```python
from build123d import *

# Parameters (mm, degrees)
SKETCH1_R           = 18.5
SKETCH1_R_2         = 11.5
BOSS_EXTRUDE1_DEPTH = 1.6
SKETCH2_W           = 5
SKETCH2_H           = 5
BOSS_EXTRUDE2_DEPTH = 1.7
CIRPATTERN1_COUNT   = 12
SKETCH3_R           = 1
CUT_EXTRUDE1_DEPTH  = 2
CIRPATTERN2_COUNT   = 2
SKETCH4_R           = 1
CUT_EXTRUDE2_DEPTH  = 10
CIRPATTERN3_COUNT   = 2


with BuildPart() as part:
    # Sketch1 → Boss-Extrude1 (new body)
    with BuildSketch(Plane.XY):
        Circle(SKETCH1_R)
        Circle(SKETCH1_R_2, mode=Mode.SUBTRACT)
    extrude(amount=BOSS_EXTRUDE1_DEPTH)

    # Sketch2 → Boss-Extrude2 (add)
    with BuildSketch(Plane.XY.offset(1.6)):
        with Locations((0, 15)):
            Rectangle(SKETCH2_W, SKETCH2_H)
    boss_extrude2 = extrude(amount=BOSS_EXTRUDE2_DEPTH)

    # CirPattern1: Boss-Extrude2 ×12 about axis
    cirpattern1_axis = Axis((0, 0, 0), (0, 0, 1))
    for i in range(1, CIRPATTERN1_COUNT):
        add(boss_extrude2.rotate(cirpattern1_axis, i * 360 / CIRPATTERN1_COUNT))

    # Sketch3 → Cut-Extrude1 (cut)
    with BuildSketch(Plane.XY.offset(1.6)):
        with Locations((-4.270514244, 15.937776134)):
            Circle(SKETCH3_R)
    cut_extrude1 = extrude(amount=-CUT_EXTRUDE1_DEPTH, mode=Mode.SUBTRACT)

    # CirPattern2: Cut-Extrude1 ×2 about axis
    cirpattern2_axis = Axis((0, 0, 0), (0, 0, 1))
    for i in range(1, CIRPATTERN2_COUNT):
        add(cut_extrude1.rotate(cirpattern2_axis, i * 360 / CIRPATTERN2_COUNT), mode=Mode.SUBTRACT)

    # Sketch4 → Cut-Extrude2 (cut)
    with BuildSketch(Plane.XY.offset(1.6)):
        with Locations((-15.937776134, 4.270514244)):
            Circle(SKETCH4_R)
    cut_extrude2 = extrude(amount=-CUT_EXTRUDE2_DEPTH, mode=Mode.SUBTRACT)

    # CirPattern3: Cut-Extrude2 ×2 about axis
    cirpattern3_axis = Axis((0, 0, 0), (0, 0, 1))
    for i in range(1, CIRPATTERN3_COUNT):
        add(cut_extrude2.rotate(cirpattern3_axis, i * 360 / CIRPATTERN3_COUNT), mode=Mode.SUBTRACT)


solid = part.part
```
Geometry: final body of the model. Coordinates: model frame, mm. A direction names the side the tool comes from. Coordinates: 2 decimals unless noted, no trailing zeros. Order: outer loops, then holes, each group sorted by start corner. A loop starts at its lowest first (then second) coordinate and runs counter-clockwise, first axis right, second up. Notation, with made-up numbers: M 65,64 L 104,64 A23 cw 104,90 Z; hole C 9,-7.5 d5. An arc over 180 degrees is marked long. Answer as CSV lines item,"result".
Q1. Draft query along Y for faces 1 (the flat face through (15, -2.5, 2)), 2 (the flat face through (5.317, 14.21, 2.438)), 3 (the flat face through (-15, -2.5, 2)), 4 (the flat face through (-7, -13, 3.3)). Return one class per face: pulls with the +Y half, pulls with the -Y half, needs draft (parallel to the pull), parting line crosses it, or undercut.
Answers:
face 1,"undercut"
face 2,"pulls with the +Y half"
face 3,"undercut"
face 4,"needs draft"
Q2. Section A-A on y = 0. Return the cut outline in (x, z), and give its area (3 significant figures).
Answers:
outline,"M -18.5,0 L -11.5,0 L -11.5,1.6 L -12.5,1.6 L -12.5,3.3 L -17.5,3.3 L -17.5,1.6 L -18.5,1.6 Z; M 11.5,0 L 18.5,0 L 18.5,1.6 L 17.5,1.6 L 17.5,3.3 L 12.5,3.3 L 12.5,1.6 L 11.5,1.6 Z"
area,"39.4 mm^2"
Q3. Set-up query: faces 5 (the flat face through (-17.5, 0, 2)), 6 (the flat face through (5.317, -14.21, 2.438)), 7 (the flat face through (-2.5, 15, 2)), 8 (the flat face through (8.78, -15.14, 2.44)), 9 (the flat face through (0, 17.5, 2)). Return all of +Z, -Z, +X, -X, +Y, -Y with unobstructed straight access to the full face (end or side cutting, diameter ignored); none if empty.
Answers:
face 5,"+Z, -X, +Y, -Y"
face 6,"+Z, -Y"
face 7,"+Z, +Y, -Y"
face 8,"+Z, +X, -Y"
face 9,"+Z, +X, -X, +Y"
Q4. Line query: probe 1 along X at (y, z) = (1.5, 2.35); probe 2 along Z at (x, y) = (5, 14). Output: solid intervals per line, ascending. Write a range as [from, to].
Answers:
probe 1,"x = [-17.5, -12.5], [12.5, 17.5]"
probe 2,"z = [0, 1.6]"
Q5. First-contact query: P1, Ø0.8, axis at x = 0.5, z = 3, coming from the -Y side; P2, Ø0.5, axis at y = 1, z = 2, coming from the +X side; P3, Ø3, axis at x = -15.94, y = 4.27, coming from the +Z side; P4, Ø1.2, axis at x = -4.27, y = 15.94, coming from the -Z side. Flat tips, straight axial feed; report the tip coordinate or a pass-through.
Answers:
P1,"stops at y = -17.5"
P2,"stops at x = 17.5"
P3,"stops at z = 1.6"
P4,"passes through"
Q6. Section C-C on x = 13. Return the cut outline in (y, z), and give its area (3 significant figures).
Answers:
outline,"M -13.16,0 L 13.16,0 L 13.16,1.6 L 10.39,1.6 L 10.39,3.3 L 4.62,3.3 L 4.62,1.6 L 2.5,1.6 L 2.5,3.3 L -2.5,3.3 L -2.5,1.6 L -4.62,1.6 L -4.62,3.3 L -10.39,3.3 L -10.39,1.6 L -13.16,1.6 Z"
area,"70.2 mm^2"
